Design review of the part built by this model. Coordinates are the model's own, in mm. A direction names the side the tool comes from. Give positions to 0.01 mm unless a question says otherwise; leave off trailing zeros. Write each loop counter-clockwise with the first axis right and the second up, starting at its lowest first coordinate (ties: lowest second). Pieces come first, ordered by that corner, then holes. Notation, with made-up numbers: M 7.25,13.5 L 16.25,13.5 A19 ccw 16.25,38.5 Z; hole C 19,-29 d4. An arc over 180 degrees is marked long. Write each question's results on one line, items separated by ' | '. Start each with the question number.
from build123d import *

# Parameters (mm, degrees)
SKETCH1_W           = 40
SKETCH1_H           = 40
BOSS_EXTRUDE1_DEPTH = 8
SKETCH6_W           = 40
SKETCH6_H           = 8
BOSS_EXTRUDE4_DEPTH = 10
BOSS_EXTRUDE2_DEPTH = 20.2
SKETCH3_W           = 40
SKETCH3_H           = 40
BOSS_EXTRUDE3_DEPTH = 10
SKETCH4_R           = 2.6
CUT_EXTRUDE1_DEPTH  = 69.258625829
SKETCH5_R           = 4.4
SKETCH5_R_2         = 2.6
CUT_EXTRUDE2_DEPTH  = 30.2
SKETCH5_3_R         = 4.4
SKETCH5_3_R_2       = 2.6
CUT_EXTRUDE3_DEPTH  = 5.5
CUT_EXTRUDE4_START  = -32.7
SKETCH5_4_R         = 4.4
SKETCH5_4_R_2       = 2.6
CUT_EXTRUDE4_DEPTH  = 5.5
SKETCH7_W           = 16.2
SKETCH7_H           = 16.2
CUT_EXTRUDE5_DEPTH  = 10
CHAMFER1_SIZE       = 0.5


with BuildPart() as part:
    # Sketch1 → Boss-Extrude1 (new body)
    with BuildSketch(Plane.XY):
        with Locations((20, 20)):
            Rectangle(SKETCH1_W, SKETCH1_H)
    extrude(amount=BOSS_EXTRUDE1_DEPTH)

    # Sketch6 → Boss-Extrude4 (add)
    with BuildSketch(Plane.XZ):
        with Locations((20, 4)):
            Rectangle(SKETCH6_W, SKETCH6_H)
    extrude(amount=BOSS_EXTRUDE4_DEPTH)

    # Sketch2 → Boss-Extrude2 (add)
    with BuildSketch(Plane.XY.offset(8)):
        Polygon((0, 40), (10, 40), (30, 40), (40, 40), (40, 0), (30.1, 0), (30.1, 35), (9.9, 35), (9.9, 0), (0, 0), align=None)
    extrude(amount=BOSS_EXTRUDE2_DEPTH)

    # Sketch3 → Boss-Extrude3 (add)
    with BuildSketch(Plane.XY.offset(28.2)):
        with Locations((20, 20)):
            Rectangle(SKETCH3_W, SKETCH3_H)
    extrude(amount=BOSS_EXTRUDE3_DEPTH)

    # Sketch4 → Cut-Extrude1 (cut, through all)
    with BuildSketch(Plane.XY.offset(38.2)):
        with Locations((35, 35)):
            Circle(SKETCH4_R)
        with Locations((35, -5)):
            Circle(SKETCH4_R)
        with Locations((5, 35)):
            Circle(SKETCH4_R)
        with Locations((5, -5)):
            Circle(SKETCH4_R)
        with Locations((20, 28)):
            Circle(SKETCH4_R)
        with Locations((20, 8)):
            Circle(SKETCH4_R)
    extrude(amount=-CUT_EXTRUDE1_DEPTH, mode=Mode.SUBTRACT)

    # Sketch5 → Cut-Extrude2 (cut)
    # profile 1 of 8: a face of its own
    with BuildSketch(Plane.XY.offset(38.2)):
        with Locations((5, 35)):
            Circle(SKETCH5_R)
        with Locations((5, 35)):
            Circle(SKETCH5_R_2, mode=Mode.SUBTRACT)
    # profile 2 of 8: a face of its own
    with BuildSketch(Plane.XY.offset(38.2)):
        with Locations((35, 35)):
            Circle(SKETCH5_R)
        with Locations((35, 35)):
            Circle(SKETCH5_R_2, mode=Mode.SUBTRACT)
    # profile 3 of 8: a face of its own
    with BuildSketch(Plane.XY.offset(38.2)):
        with Locations((35, -5)):
            Circle(SKETCH5_R)
    # profile 4 of 8: a face of its own
    with BuildSketch(Plane.XY.offset(38.2)):
        with Locations((5, -5)):
            Circle(SKETCH5_R)
    # profile 5 of 8: a face of its own
    with BuildSketch(Plane.XY.offset(38.2)):
        with BuildLine():
            ThreePointArc((5, 30.6), (1.888730163, 38.111269837), (9.4, 35))
            Line((9.4, 35), (9.4, 40))
            Line((9.4, 40), (0, 40))
            Line((0, 40), (0, 30.6))
            Line((0, 30.6), (5, 30.6))
        make_face()
    # profile 6 of 8: a face of its own
    with BuildSketch(Plane.XY.offset(38.2)):
        with BuildLine():
            Line((40, 40), (30.6, 40))
            Line((30.6, 40), (30.6, 35))
            ThreePointArc((30.6, 35), (35, 39.4), (39.4, 35))
            ThreePointArc((39.4, 35), (38.111269837, 31.888730163), (35, 30.6))
            Line((35, 30.6), (40, 30.6))
            Line((40, 30.6), (40, 40))
        make_face()
    # profile 7 of 8: a face of its own
    with BuildSketch(Plane.XY.offset(38.2)):
        with Locations((35, -5)):
            Circle(SKETCH5_R)
    # profile 8 of 8: a face of its own
    with BuildSketch(Plane.XY.offset(38.2)):
        with Locations((5, -5)):
            Circle(SKETCH5_R)
    extrude(amount=-CUT_EXTRUDE2_DEPTH, mode=Mode.SUBTRACT)

    # Sketch5<3> → Cut-Extrude3 (cut)
    # profile 1 of 2: a face of its own
    with BuildSketch(Plane.XY.offset(38.2)):
        with Locations((20, 28)):
            Circle(SKETCH5_3_R)
        with Locations((20, 28)):
            Circle(SKETCH5_3_R_2, mode=Mode.SUBTRACT)
    # profile 2 of 2: a face of its own
    with BuildSketch(Plane.XY.offset(38.2)):
        with Locations((20, 8)):
            Circle(SKETCH5_3_R)
        with Locations((20, 8)):
            Circle(SKETCH5_3_R_2, mode=Mode.SUBTRACT)
    extrude(amount=-CUT_EXTRUDE3_DEPTH, mode=Mode.SUBTRACT)

    # Sketch5<4> → Cut-Extrude4 (cut)
    # profile 1 of 2: a face of its own
    with BuildSketch(Plane.XY.offset(38.2).offset(CUT_EXTRUDE4_START)):
        with Locations((20, 28)):
            Circle(SKETCH5_4_R)
        with Locations(Location((20, 28, 0), (0, 0, 180))):
            Circle(SKETCH5_4_R_2, mode=Mode.SUBTRACT)
    # profile 2 of 2: a face of its own
    with BuildSketch(Plane.XY.offset(38.2).offset(CUT_EXTRUDE4_START)):
        with Locations((20, 8)):
            Circle(SKETCH5_4_R)
        with Locations(Location((20, 8, 0), (0, 0, 180))):
            Circle(SKETCH5_4_R_2, mode=Mode.SUBTRACT)
    extrude(amount=-CUT_EXTRUDE4_DEPTH, mode=Mode.SUBTRACT)

    # Sketch7 → Cut-Extrude5 (cut)
    with BuildSketch(Plane.XZ.offset(-35)):
        with Locations((20, 18.1)):
            Rectangle(SKETCH7_W, SKETCH7_H)
    extrude(amount=-CUT_EXTRUDE5_DEPTH, mode=Mode.SUBTRACT)

    # Chamfer1
    chamfer1_edges = [part.edges().sort_by_distance(p)[0] for p in [
        (9.9, 0, 18.1),
        (30.1, 0, 18.1),
        (20, 0, 28.2),
    ]]
    chamfer(chamfer1_edges, length=CHAMFER1_SIZE)


solid = part.part
Q1. Wall thickness on line 1 along Y through (x, z) = (35, 4.75); line 2 along Y through (x, z) = (20, 1); line 3 along X through (y, z) = (8, 7.25): over which ranges is each line inside the solid? List them lowest first. Write a range as from..to.
Q2. We need section D-D on z = 7. Write out the cut boundary in (x, y), and give its area (3 significant figures).
Q3. We need section C-C on x = 25. Write out the cut boundary in (y, z), and give its area (3 significant figures).
Q4. For pin 1 Ø4 at (x, z) = (27.5, 32) entering from -Y; pin 2 Ø4 at (x, z) = (3.5, 25) entering from +Y; pin 3 Ø10 at (x, z) = (4.5, 13.5) entering from +Y; pin 4 Ø1.5 at (y, z) = (37.5, 17.5) entering from +X, all flat-tipped, find the tip position at first contact; note any pin that passes through.
Q5. The part is to be moulded in two halves that separate along X. For faces 6 (the flat face through (11, 35, 18)), 7 (the flat face through (20, 20, 38.2)), 8 (the flat face through (40, 15, 15)), 9 (the cylindrical face through (22.4, 7, 6.8)), say which applies: pulls with the +X half, pulls with the -X half, needs draft (parallel to the pull), parting line crosses it, or undercut.
Q6. We need section A-A on y = 8. Write out the cut boundary in (x, z), and give its area (3 significant figures).
Q7. For faces 1 (the flat face through (11.9, 37, 18)), 2 (the cylindrical face through (15.604, 8.193, 2.788)), 3 (the flat face through (36.3, 37.5, 8)), 4 (the cylindrical face through (16.757, 30.974, 35.488)), 5 (the flat face through (30.1, 18, 18)), list the 3-axis set-ups (+Z, -Z, +X, -X, +Y, -Y) from which the entire face can be reached by the end or side of a thin tool; tool diameter is ignored.
Q8. We need section B-B on z = 18.5. Write out the cut boundary in (x, y).
Answer sheet:
1) line 1: -10..-7.6, -2.4..32.4, 37.6..40 | line 2: -10..3.6, 12.4..23.6, 32.4..40 | line 3: 0..17.4, 22.6..40
2) outline: M 0,-10 L 40,-10 L 40,40 L 0,40 Z; hole C 5,-5 d5.2; hole C 5,35 d5.2; hole C 20,8 d5.2; hole C 20,28 d5.2; hole C 35,-5 d5.2; hole C 35,35 d5.2 | area: 1,870 mm^2
3) outline: M -10,0 L 40,0 L 40,10 L 35,10 L 35,8 L -10,8 Z; M 0,28.7 L 0.5,28.2 L 35,28.2 L 35,26.2 L 40,26.2 L 40,38.2 L 0,38.2 Z | area: 820 mm^2
4) pin 1: y = 0 | pin 2: y = 30.63 | pin 3: y = 40 | pin 4: x = 30.6
5) face 6: undercut | face 7: needs draft | face 8: pulls with the +X half | face 9: undercut
6) outline: M 0,0 L 15.6,0 L 15.6,5.5 L 17.4,5.5 L 17.4,8 L 9.9,8 L 9.9,28.2 L 17.4,28.2 L 17.4,32.7 L 15.6,32.7 L 15.6,38.2 L 0,38.2 Z; M 22.6,5.5 L 24.4,5.5 L 24.4,0 L 40,0 L 40,38.2 L 24.4,38.2 L 24.4,32.7 L 22.6,32.7 L 22.6,28.2 L 30.1,28.2 L 30.1,8 L 22.6,8 Z | area: 987 mm^2
7) face 1: +Y, -Y | face 2: -Z | face 3: +Z, +X, +Y | face 4: +Z | face 5: -Y
8) outline: M 0,0 L 9.4,0 L 9.9,0.5 L 9.9,35 L 11.9,35 L 11.9,40 L 9.4,40 L 9.4,35 A4.4 cw 5,30.6 L 0,30.6 Z; M 28.1,35 L 30.1,35 L 30.1,0.5 L 30.6,0 L 40,0 L 40,30.6 L 35,30.6 A4.4 cw 30.6,35 L 30.6,40 L 28.1,40 Z
